from build123d import *

# Parameters (mm, degrees)
BOSS_EXTRUDE1_DEPTH = 0.1
SKETCH2_R           = 0.2
BOSS_EXTRUDE2_DEPTH = 1
SKETCH3_R           = 3
BOSS_EXTRUDE3_DEPTH = 0.3
SKETCH4_R           = 0.15
CUT_EXTRUDE1_DEPTH  = 2.3


with BuildPart() as part:
    # Sketch1 → Boss-Extrude1 (new body)
    with BuildSketch(Plane(origin=(0, 0, 0), x_dir=(1, 0, 0), z_dir=(0, 1, 0))):
        with BuildLine():
            Line((-0.25, 8.545435606), (0.25, 8.545435606))
            Line((0.25, 8.545435606), (0.25, 0.601234649))
            ThreePointArc((0.25, 0.601234649), (0, -0.651139849), (-0.25, 0.601234649))
            Line((-0.25, 0.601234649), (-0.25, 8.545435606))
        make_face()
    extrude(amount=BOSS_EXTRUDE1_DEPTH)

    # Sketch2 → Boss-Extrude2 (add)
    with BuildSketch(Plane.XZ.offset(-0.1)):
        Circle(SKETCH2_R)
    extrude(amount=BOSS_EXTRUDE2_DEPTH)

    # Sketch3 → Boss-Extrude3 (add)
    with BuildSketch(Plane.XZ.offset(0.9)):
        Circle(SKETCH3_R)
    extrude(amount=BOSS_EXTRUDE3_DEPTH)

    # Sketch4 → Cut-Extrude1 (cut, through all)
    with BuildSketch(Plane(origin=(0, 0.1, 0), x_dir=(1, 0, 0), z_dir=(0, 1, 0))):
        Circle(SKETCH4_R)
    extrude(amount=-CUT_EXTRUDE1_DEPTH, mode=Mode.SUBTRACT)


solid = part.part
Verification items for the finished model (mm, model axes). Round coordinates to 2 decimals unless told otherwise and drop trailing zeros. Loops run counter-clockwise (first coordinate to the right, second up) from the corner with the lowest first, then second, coordinate; pieces in that order, holes last. Notation, with made-up numbers: M 13,77 L 37,77 A35 ccw 37,116 Z; hole C 68.5,71.5 d11. An arc over 180 degrees is marked long. Write each question's results on one line, items separated by ' | '.
1) Scan lines: L1, parallel to Y at x = -1.65, z = 0.5; L2, parallel to Z at x = -1.1, y = -1.1; L3, parallel to Z at x = 1.7, y = -1. Record each from-to range of solid material in increasing order. Write a range as from..to.
Checks:
L1: y = -1.2..-0.9 | L2: z = -2.79..2.79 | L3: z = -2.47..2.47
2) Section check C-C on y = -0.7. Record the boundary of the cut face in (x, z).
Checks:
outline: C 0,0 d0.4; hole C 0,0 d0.3
3) Section check B-B on z = -1.25. Record the boundary of the cut face in (x, y), then the cut area to 3 significant figures.
Checks:
outline: M -2.73,-1.2 L 2.73,-1.2 L 2.73,-0.9 L -2.73,-0.9 Z; M -0.25,0 L 0.25,0 L 0.25,0.1 L -0.25,0.1 Z | area: 1.69 mm2
4) Section check A-A on x = 0. Record the boundary of the cut face in (y, z), then the cut area to 3 significant figures.
Checks:
outline: M -1.2,-3 L -0.9,-3 L -0.9,-0.2 L 0,-0.2 L 0,-8.55 L 0.1,-8.55 L 0.1,-0.15 L -1.2,-0.15 Z; M -1.2,0.15 L 0.1,0.15 L 0.1,0.65 L 0,0.65 L 0,0.2 L -0.9,0.2 L -0.9,3 L -1.2,3 Z | area: 2.69 mm2
5) Section check D-D on z = 0. Record the boundary of the cut face in (x, y), then the cut area to 3 significant figures.
Checks:
outline: M -3,-1.2 L -0.15,-1.2 L -0.15,0.1 L -0.65,0.1 L -0.65,0 L -0.2,0 L -0.2,-0.9 L -3,-0.9 Z; M 0.15,-1.2 L 3,-1.2 L 3,-0.9 L 0.2,-0.9 L 0.2,0 L 0.65,0 L 0.65,0.1 L 0.15,0.1 Z | area: 1.90 mm2
